For this review, use the dimensioned drawing (mm, ordinates from the lowest corner) and the shaded views. A direction names the side the tool comes from. Give positions to 0.01 mm unless a question says otherwise; leave off trailing zeros. Order: outer loops, then holes, each group sorted by start corner. A loop starts at its lowest first (then second) coordinate and runs counter-clockwise, first axis right, second up. Notation, with made-up numbers: (-34.5, -18.75) - (0.5, -18.75) arc R14 ccw to (0.5, 3.25) - close; hole circle Ø7 at (74.25, -9.5). An arc over 180 degrees is marked (long way). Use a Markdown table: item, result. Add a question column.
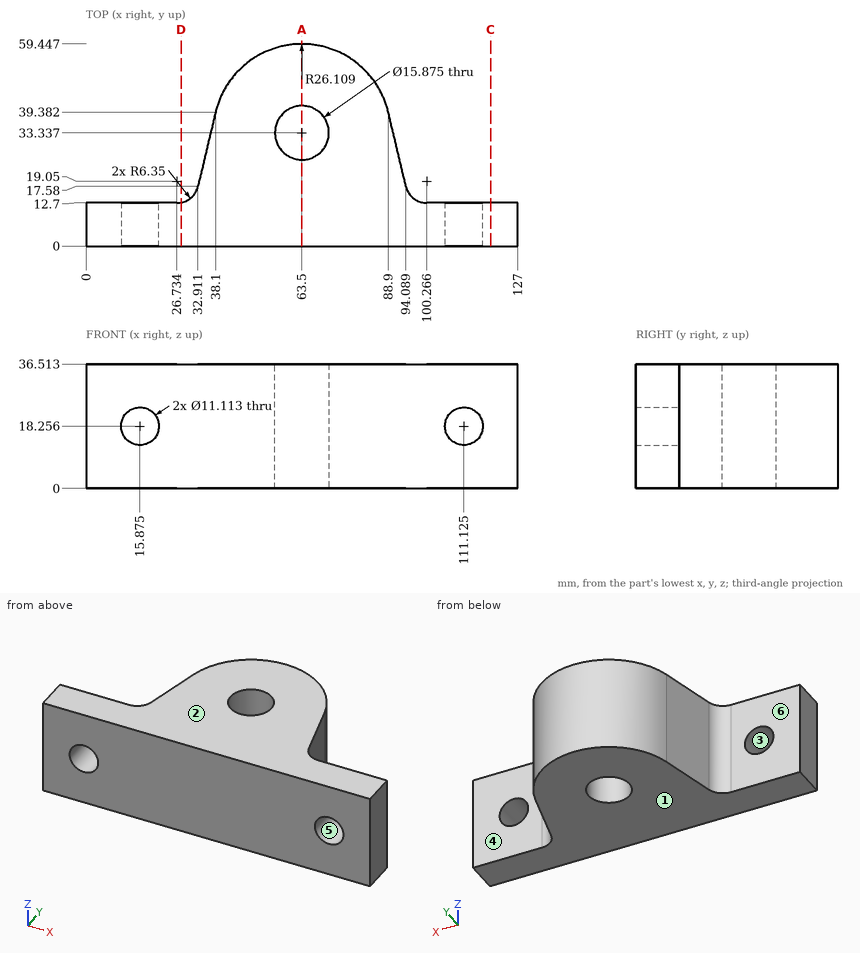
Q1. Draft analysis for pull direction Z (two halves, no side actions). For the marked faces 1, 2, 3 and 4, state which applies: pulls with the +Z half, pulls with the -Z half, needs draft (parallel to the pull), parting line crosses it, or undercut.
Q2. We need section D-D (x = 28). Write out the cut boundary in (y, z).
Q3. Wall thickness on probe 1 along Y at (x, z) = (120, 27.5); probe 2 along Y at (x, z) = (86.5, 9) (1 decimal); probe 3 along X at (y, z) = (37.5, 24): over which ranges is each line inside the solid? List them lowest first.
Q4. We need section A-A (x = 63.5). Write out the cut boundary in (y, z) (1 decimal), plus the area to 3 significant figures.
Q5. Machinability: for the marked faces 5 and 6, which of the approach directions +Z, -Z, +X, -X, +Y, -Y give a long, thin tool a straight path to every point of the face, cutting with its end or side? Answer none if there is none.
Q6. Clearance check with flat-ended pins moving along their axes: P1, Ø8, axis at x = 48.5, z = 29.5, coming from the +Y side; P2, Ø1, axis at x = 69, z = 27.5, coming from the -Y side; P3, Ø10, axis at x = 16.5, z = 29.5, coming from the +Y side; P4, Ø5, axis at y = 36.5, z = 3.5, coming from the +X side. State where each tip first meets the part, or that it passes through.
Q7. We need section C-C (x = 119). Write out the cut boundary in (y, z).
Here are the results:
| question | item | result |
|---|---|---|
| 1 | face 1 | pulls with the -Z half |
| 1 | face 2 | pulls with the +Z half |
| 1 | face 3 | undercut |
| 1 | face 4 | needs draft |
| 2 | outline | (0, 0) - (12.83, 0) - (12.83, 36.51) - (0, 36.51) - close |
| 3 | probe 1 | 0 to 12.7 |
| 3 | probe 2 | 0 to 45.7 |
| 3 | probe 3 | 37.65 to 56.74, 70.26 to 89.35 |
| 4 | outline | (0, 0) - (25.4, 0) - (25.4, 36.5) - (0, 36.5) - close; (41.3, 0) - (59.4, 0) - (59.4, 36.5) - (41.3, 36.5) - close |
| 4 | area | 1,590 mm2 |
| 5 | face 5 | +Y, -Y |
| 5 | face 6 | +Z, -Z, -X, +Y |
| 6 | P1 | y = 57.02 |
| 6 | P2 | y = 0 |
| 6 | P3 | y = 12.7 |
| 6 | P4 | x = 90.18 |
| 7 | outline | (0, 0) - (12.7, 0) - (12.7, 36.51) - (0, 36.51) - close |
